```python
from build123d import *

# Parameters (mm, degrees)
SKETCH1_W                                    = 50
SKETCH1_H                                    = 15
BOSS_EXTRUDE1_DEPTH                          = 10
CBORE_FOR_M3_HEX_SOCKET_HEAD_CAP_SCR_2_COUNT = 2
CBORE_FOR_M3_HEX_SOCKET_HEAD_CAP_SCR_2_PITCH = 24


with BuildPart() as part:
    # Sketch1 → Boss-Extrude1 (new body)
    with BuildSketch(Plane.XY):
        with Locations((6, 9.5)):
            Rectangle(SKETCH1_W, SKETCH1_H)
    extrude(amount=BOSS_EXTRUDE1_DEPTH)

    # Sketch2 → Cut-Revolve1 (revolve, cut)
    with BuildSketch(Plane(origin=(0, 0, 0), x_dir=(0, 0, -1), z_dir=(1, 0, 0))):
        Polygon((0, 17), (-7, 17), (-7, 15.5), (-8, 15.5), (-8, 11.8), (-6, 11.8), (-6, 5.8), (-8, 5.8), (-8, 2.8), (-6.25, 2.8), (-6.25, 2), (0, 2), align=None)
    revolve(axis=Axis((0, 2, 0), (0, 1, 0)), mode=Mode.SUBTRACT)

    # Sketch4 → CBORE for M3 Hex Socket Head Cap Screw1 (revolve, cut)
    with BuildSketch(Plane(origin=(-12, 8.8, 10), x_dir=(0, -1, 0), z_dir=(1, 0, 0))):
        Polygon((0, 0), (0, 10), (1.7, 10), (1.7, 3.4), (3.25, 3.4), (3.25, 0.025), (3.275, 0), align=None)
    cbore_for_m3_hex_socket_head_cap_screw1 = revolve(axis=Axis((-12, 8.8, 16.35), (0, 0, -1)), mode=Mode.SUBTRACT)

    # CBORE for M3 Hex Socket Head Cap Scr 2: CBORE for M3 Hex Socket Head Cap Screw1 ×2
    with Locations(*[(i * CBORE_FOR_M3_HEX_SOCKET_HEAD_CAP_SCR_2_PITCH, 0, 0) for i in range(1, CBORE_FOR_M3_HEX_SOCKET_HEAD_CAP_SCR_2_COUNT)]):
        add(cbore_for_m3_hex_socket_head_cap_screw1, mode=Mode.SUBTRACT)


solid = part.part
```
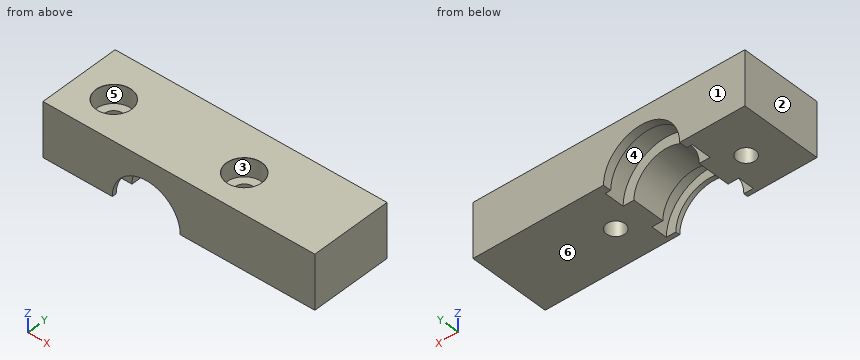
Source: CAD feature listing. Evaluate the final solid. Frame: model axes, mm. Face numbers are marked on the shaded views. A direction names the side the tool comes from. Round coordinates to 2 decimals unless told otherwise and drop trailing zeros. Loops run counter-clockwise (first coordinate to the right, second up) from the corner with the lowest first, then second, coordinate; pieces in that order, holes last.
(1) Section query A-A (y = 8.8). Output: boundary loops of the cut face in (x, z) (3 decimals), and give its area (3 significant figures).
From the geometry:
outline: (-19, 0) - (-13.7, 0) - (-13.7, 6.6) - (-15.25, 6.6) - (-15.25, 9.975) - (-15.275, 10) - (-19, 10) - close; (-10.3, 0) - (-6, 0) arc R6 cw to (6, 0) - (10.3, 0) - (10.3, 6.6) - (8.75, 6.6) - (8.75, 9.975) - (8.725, 10) - (-8.725, 10) - (-8.75, 9.975) - (-8.75, 6.6) - (-10.3, 6.6) - close; (13.7, 0) - (31, 0) - (31, 10) - (15.275, 10) - (15.25, 9.975) - (15.25, 6.6) - (13.7, 6.6) - close
area: 354 mm2
(2) Section query B-B (x = 12). Output: boundary loops of the cut face in (y, z) (3 decimals).
From the geometry:
outline: (2, 0) - (7.1, 0) - (7.1, 6.6) - (5.55, 6.6) - (5.55, 9.975) - (5.525, 10) - (2, 10) - close; (10.5, 0) - (17, 0) - (17, 10) - (12.075, 10) - (12.05, 9.975) - (12.05, 6.6) - (10.5, 6.6) - close
(3) Section query C-C (z = 4.75). Output: boundary loops of the cut face in (x, y), and give its area (3 significant figures).
From the geometry:
outline: (-19, 2) - (-4.06, 2) - (-4.06, 2.8) - (-6.44, 2.8) - (-6.44, 5.8) - (-3.67, 5.8) - (-3.67, 11.8) - (-6.44, 11.8) - (-6.44, 15.5) - (-5.14, 15.5) - (-5.14, 17) - (-19, 17) - close; (3.67, 5.8) - (6.44, 5.8) - (6.44, 2.8) - (4.06, 2.8) - (4.06, 2) - (31, 2) - (31, 17) - (5.14, 17) - (5.14, 15.5) - (6.44, 15.5) - (6.44, 11.8) - (3.67, 11.8) - close; hole circle Ø3.4 at (-12, 8.8); hole circle Ø3.4 at (12, 8.8)
area: 580 mm2
(4) Pull-direction query (X, two-part tool) for the marked faces 1, 2 and 3; classes: +X half, -X half, draft (parallel to the pull), parting line (faces both ways), or undercut.
From the geometry:
face 1: draft
face 2: -X half
face 3: undercut
(5) Material intervals for probe 1 along X at (y, z) = (8.8, 8.9); probe 2 along Y at (x, z) = (-12, 1.75); probe 3 along X at (y, z) = (8.8, 4.75), sorted ascending.
From the geometry:
probe 1: x = -19 to -15.25, -8.75 to 8.75, 15.25 to 31
probe 2: y = 2 to 7.1, 10.5 to 17
probe 3: x = -19 to -13.7, -10.3 to -3.67, 3.67 to 10.3, 13.7 to 31
(6) Access query for the marked faces 4, 5 and 6. Directions: +Z, -Z, +X, -X, +Y, -Y. A direction counts if a zero-diameter tool reaches every point of the face in a straight line with its end or side. Return the directions, or none.
From the geometry:
face 4: -Z
face 5: +Z
face 6: -Z, +X, -X, +Y, -Y
(7) Section query D-D (x = 0). Output: boundary loops of the cut face in (y, z).
From the geometry:
outline: (2, 6.25) - (2.8, 6.25) - (2.8, 8) - (5.8, 8) - (5.8, 6) - (11.8, 6) - (11.8, 8) - (15.5, 8) - (15.5, 7) - (17, 7) - (17, 10) - (2, 10) - close
(8) Contact query for flat-ended pins moving along their axis: pin 1 Ø5.5 at (x, y) = (12, 8.8) entering from +Z; pin 2 Ø2.5 at (x, z) = (3, 4) entering from +Y. Output: stop coordinate, or through.
From the geometry:
pin 1: stops at z = 6.6
pin 2: stops at y = 11.8
